Autodesk Inventor part; units mm, degrees
ref_plane "YZ Plane" through (0, 0, 0) normal (1, 0, 0) x (0, 1, 0)
ref_plane "XZ Plane" through (0, 0, 0) normal (0, 1, 0) x (-1, 0, 0)
ref_plane "XY Plane" through (0, 0, 0) normal (0, 0, 1) x (1, 0, 0)
sketch "Sketch1" plane through (0, 0, 0) normal (0, 1, 0) x (-1, 0, 0)
  line L0 (-9.4777, 15.0257) -> (40.5223, 15.0257)
  line L1 (40.5223, 15.0257) -> (40.5223, -84.9743)
  line L2 (40.5223, -84.9743) -> (-9.4777, -84.9743)
  line L3 (-9.4777, -84.9743) -> (-9.4777, 15.0257)
  line L4 (35.5223, 10.0257) -> (-4.4777, 10.0257)
  line L5 (-4.4777, 10.0257) -> (-4.4777, -79.9743)
  line L6 (-4.4777, -79.9743) -> (35.5223, -79.9743)
  line L7 (35.5223, -79.9743) -> (35.5223, 10.0257)
  point P0 (0, 0)
  dimension "d0" = 50
  dimension "d1" = 100
  dimension "d2" = 5
  dimension "d3" = 90
  dimension "d4" = 5
  dimension "d5" = 40
extrude "Extrusion1" add sketch "Sketch1" along normal blind 800
sketch "Sketch3" plane through (-40.5223, 0, 15.0257) normal (0, 0, 1) x (1, 0, 0)
  line L0 (0, 0) -> (0, 800)
  line L1 (0, 800) -> (50, 750)
  line L2 (0, 800) -> (70.7107, 800) construction
  line L3 (50, 800) -> (0, 800)
  line L4 (0, 800) -> (50, 800)
  line L5 (50, 800) -> (50, 750)
  line L6 (50, 0) -> (50, 800)
  point P0 (40.5223, 0)
  dimension "d8" = 45
extrude "Extrusion2" cut sketch "Sketch3" against normal blind 800
properties part number "PerfilV1"
The listing builds one solid part. Answer for the finished solid, in the listing's coordinates (mm). A direction names the side the tool comes from. Give positions to 0.01 mm unless a question says otherwise; leave off trailing zeros. Write each loop counter-clockwise with the first axis right and the second up, starting at its lowest first coordinate (ties: lowest second). Pieces come first, ordered by that corner, then holes.
Item 1: Determine the mould class of faces 1 (the flat face through (9.478, 370, -36)), 2 (the flat face through (-15, 392, -79.974)), 3 (the flat face through (-16, 394, -84.974)) for opening direction X: released by +X, released by -X, zero draft, split by the parting line, or undercut.
Item 2: Section B-B, the plane x = -14.5 is taken. Write down the section's boundary in (y, z), plus the area to 3 significant figures.
Item 3: Section A-A, the plane z = -1.5 is taken. Write down the section's boundary in (x, y).
Item 4: Section C-C, the plane y = 367.5 is taken. Write down the section's boundary in (x, z), plus the area to 3 significant figures.
Item 5: Find the intervals of material crossed by line 1 along Z through (x, y) = (-16, 251); line 2 along X through (y, z) = (71, -18); line 3 along X through (y, z) = (761, -73), in increasing order.
Item 6: Which of the six approach directions +Z, -Z, +X, -X, +Y, -Y give full straight-line access (tool end or side, diameter ignored) to faces 4 (the flat face through (-15, 394, 15.026)), 5 (the flat face through (-16, 392, 10.026))?
Completed:
1. face 1: released by +X
1. face 2: undercut
1. face 3: zero draft
2. outline: (0, -84.97) - (773.98, -84.97) - (773.98, -79.97) - (0, -79.97) - close; (0, 10.03) - (773.98, 10.03) - (773.98, 15.03) - (0, 15.03) - close
2. area: 7,740 mm2
3. outline: (-40.52, 0) - (-35.52, 0) - (-35.52, 795) - (-40.52, 800) - close; (4.48, 0) - (9.48, 0) - (9.48, 750) - (4.48, 755) - close
4. outline: (-40.52, -84.97) - (9.48, -84.97) - (9.48, 15.03) - (-40.52, 15.03) - close; hole (-35.52, -79.97) - (4.48, -79.97) - (4.48, 10.03) - (-35.52, 10.03) - close
4. area: 1,400 mm2
5. line 1: z = -84.97 to -79.97, 10.03 to 15.03
5. line 2: x = -40.52 to -35.52, 4.48 to 9.48
5. line 3: x = -40.52 to -35.52
6. face 4: +Z, +X, -X, +Y, -Y
6. face 5: +Y, -Y
